Geometry check sheet. Reference: the model listing, model coordinates, mm. Face numbers are marked on the shaded views. A direction names the side the tool comes from. Coordinates: 2 decimals unless noted, no trailing zeros. Loops run counter-clockwise (first coordinate to the right, second up) from the corner with the lowest first, then second, coordinate; pieces in that order, holes last. Notation, with made-up numbers: M -9,-37.5 L 42,-37.5 A27 cw 42,-12.5 Z; hole C 15.5,54 d1. An arc over 180 degrees is marked long. Use CSV: the item, a comma, the result in double quotes.
Autodesk Inventor part; units mm, degrees
ref_plane "YZ Plane" through (0, 0, 0) normal (1, 0, 0) x (0, 1, 0)
ref_plane "XZ Plane" through (0, 0, 0) normal (0, 1, 0) x (-1, 0, 0)
ref_plane "XY Plane" through (0, 0, 0) normal (0, 0, 1) x (1, 0, 0)
sketch "Sketch1" plane through (0, 0, 0) normal (0, 0, 1) x (1, 0, 0)
  line L0 (0, 0) -> (22, 0)
  line L1 (22, 0) -> (22, -29)
  line L2 (22, -29) -> (0, -29)
  line L3 (0, -29) -> (0, 0)
  line L4 (3, -5.35) -> (19, -5.35)
  line L5 (19, -5.35) -> (19, -7.65)
  line L6 (19, -7.65) -> (3, -7.65)
  line L7 (3, -7.65) -> (3, -5.35)
  line L8 (3, -13.35) -> (19, -13.35)
  line L9 (19, -13.35) -> (19, -15.65)
  line L10 (19, -15.65) -> (3, -15.65)
  line L11 (3, -15.65) -> (3, -13.35)
  line L12 (3, -21.35) -> (19, -21.35)
  line L13 (19, -21.35) -> (19, -23.65)
  line L14 (19, -23.65) -> (3, -23.65)
  line L15 (3, -23.65) -> (3, -21.35)
  line L16 (19, -5.35) -> (19, -13.35) construction
  line L17 (19, -13.35) -> (19, -21.35) construction
  line L18 (22, -14.5) -> (0, -14.5) construction
  line L19 (11, 0) -> (11, -29) construction
  point P0 (19, -14.5)
  point P1 (11, -5.35)
  dimension "d0" = 22
  dimension "d1" = 29
  dimension "d2" = 2.3
  dimension "d3" = 8
  dimension "d4" = 16
extrude "Body with light pipe slots" add sketch "Sketch1" along normal blind 4.5
sketch "Sketch2" plane through (0, 0, 4.5) normal (0, 0, 1) x (1, 0, 0)
  line L0 (0, -29) -> (22, -29) construction
  line L1 (22, -29) -> (22, 0) construction
  line L2 (22, 0) -> (0, 0) construction
  line L3 (0, 0) -> (0, -29) construction
  line L4 (3, -21.35) -> (19, -21.35) construction
  line L5 (19, -21.35) -> (19, -23.65) construction
  line L6 (19, -23.65) -> (3, -23.65) construction
  line L7 (3, -23.65) -> (3, -21.35) construction
  line L8 (3, -13.35) -> (19, -13.35) construction
  line L9 (19, -13.35) -> (19, -15.65) construction
  line L10 (19, -15.65) -> (3, -15.65) construction
  line L11 (3, -15.65) -> (3, -13.35) construction
  line L12 (3, -5.35) -> (19, -5.35) construction
  line L13 (19, -5.35) -> (19, -7.65) construction
  line L14 (19, -7.65) -> (3, -7.65) construction
  line L15 (3, -7.65) -> (3, -5.35) construction
  line L16 (1, -5.35) -> (21, -5.35)
  line L17 (21, -5.35) -> (21, -7.65)
  line L18 (21, -7.65) -> (1, -7.65)
  line L19 (1, -7.65) -> (1, -5.35)
  line L20 (1, -13.35) -> (21, -13.35)
  line L21 (21, -13.35) -> (21, -15.65)
  line L22 (21, -15.65) -> (1, -15.65)
  line L23 (1, -15.65) -> (1, -13.35)
  line L24 (1, -21.35) -> (21, -21.35)
  line L25 (21, -21.35) -> (21, -23.65)
  line L26 (21, -23.65) -> (1, -23.65)
  line L27 (1, -23.65) -> (1, -21.35)
  dimension "d7" = 2
  dimension "d8" = 2
extrude "Light pipe wing cuts" cut sketch "Sketch2" against normal blind 4
sketch "Sketch3" plane through (0, 0, 4.5) normal (0, 0, 1) x (1, 0, 0)
  line L0 (1, -21.35) -> (21, -21.35) construction
  line L1 (21, -21.35) -> (21, -23.65) construction
  line L2 (21, -23.65) -> (1, -23.65) construction
  line L3 (1, -23.65) -> (1, -21.35) construction
  line L4 (1, -13.35) -> (21, -13.35) construction
  line L5 (21, -13.35) -> (21, -15.65) construction
  line L6 (21, -15.65) -> (1, -15.65) construction
  line L7 (1, -15.65) -> (1, -13.35) construction
  line L8 (1, -5.35) -> (21, -5.35) construction
  line L9 (21, -5.35) -> (21, -7.65) construction
  line L10 (21, -7.65) -> (1, -7.65) construction
  line L11 (1, -7.65) -> (1, -5.35) construction
  line L12 (0, -29) -> (22, -29) construction
  line L13 (22, -29) -> (22, 0) construction
  line L14 (22, 0) -> (0, 0) construction
  line L15 (0, 0) -> (0, -29) construction
  line L16 (3, -5.35) -> (3, -7.65) construction
  line L17 (19, -7.65) -> (19, -5.35) construction
  line L18 (19, -15.65) -> (19, -13.35) construction
  line L19 (19, -23.65) -> (19, -21.35) construction
  line L20 (3, -21.35) -> (3, -23.65) construction
  line L21 (3, -13.35) -> (3, -15.65) construction
  line L22 (3, -4.35) -> (19, -4.35)
  line L23 (19, -4.35) -> (19, -8.65)
  line L24 (19, -8.65) -> (3, -8.65)
  line L25 (3, -8.65) -> (3, -4.35)
  line L26 (3, -12.35) -> (19, -12.35)
  line L27 (19, -12.35) -> (19, -16.65)
  line L28 (19, -16.65) -> (3, -16.65)
  line L29 (3, -16.65) -> (3, -12.35)
  line L30 (3, -20.2545) -> (19, -20.2545)
  line L31 (19, -20.2545) -> (19, -24.5545)
  line L32 (19, -24.5545) -> (3, -24.5545)
  line L33 (3, -24.5545) -> (3, -20.2545)
  dimension "d11" = 1
  dimension "d12" = 1
  dimension "d13" = 1.0956
  dimension "d14" = 1
extrude "SMD clearance cuts" cut sketch "Sketch3" against normal blind 1
sketch "Sketch4" plane through (0, 0, 0) normal (0, 0, -1) x (-1, 0, 0)
  line L0 (-22, 0) -> (0, 0) construction
  line L1 (-11, 0) -> (-11, -29) construction
  line L2 (0, -29) -> (-22, -29) construction
  line L3 (-12, -2.15) -> (-10, -2.15)
  line L4 (-10, -26.85) -> (-12, -26.85)
  line L5 (-3, -5.35) -> (-19, -5.35)
  line L6 (-19, -23.65) -> (-3, -23.65)
  line L7 (-6.75, -23.65) -> (-6.75, -25.15)
  line L8 (-15.25, -25.15) -> (-15.25, -23.65)
  line L9 (-19, -15.65) -> (-3, -15.65)
  line L10 (-6.75, -15.65) -> (-6.75, -17.15)
  line L11 (-15.25, -17.15) -> (-15.25, -15.65)
  line L12 (-3, -7.65) -> (-19, -7.65)
  line L13 (-6.75, -7.65) -> (-6.75, -9.15)
  line L14 (-15.25, -9.15) -> (-15.25, -7.65)
  line L15 (-12, -7.65) -> (-12, -2.15)
  line L16 (-10, -2.15) -> (-10, -7.65)
  line L17 (-6.75, -9.15) -> (-10, -9.15)
  line L18 (-12, -9.15) -> (-15.25, -9.15)
  line L19 (-12, -15.65) -> (-12, -9.15)
  line L20 (-10, -9.15) -> (-10, -15.65)
  line L21 (-15.25, -15.65) -> (-12, -15.65)
  line L22 (-10, -15.65) -> (-6.75, -15.65)
  line L23 (-6.75, -17.15) -> (-10, -17.15)
  line L24 (-12, -17.15) -> (-15.25, -17.15)
  line L25 (-15.25, -23.65) -> (-12, -23.65)
  line L26 (-10, -23.65) -> (-6.75, -23.65)
  line L27 (-6.75, -25.15) -> (-10, -25.15)
  line L28 (-12, -25.15) -> (-15.25, -25.15)
  line L29 (-12, -26.85) -> (-12, -25.15)
  line L30 (-12, -23.65) -> (-12, -17.15)
  line L31 (-10, -17.15) -> (-10, -23.65)
  line L32 (-10, -25.15) -> (-10, -26.85)
  line L33 (-15.25, -7.65) -> (-12, -7.65)
  line L34 (-10, -7.65) -> (-6.75, -7.65)
  point P0 (-11, -2.15)
  dimension "d17" = 3.2
  dimension "d18" = 2
  dimension "d19" = 3.2
  dimension "d20" = 1.5
  dimension "d21" = 8.5
  dimension "d22" = 4.25
extrude "Case interior molding cuts" cut sketch "Sketch4" against normal blind 3
equation "\"d8\" = d7"
equation "\"d12\" = d11"
equation "\"d14\" = d11"
equation "\"d22\" = 0.5 * d21"
properties part number "Lightpipe shield"
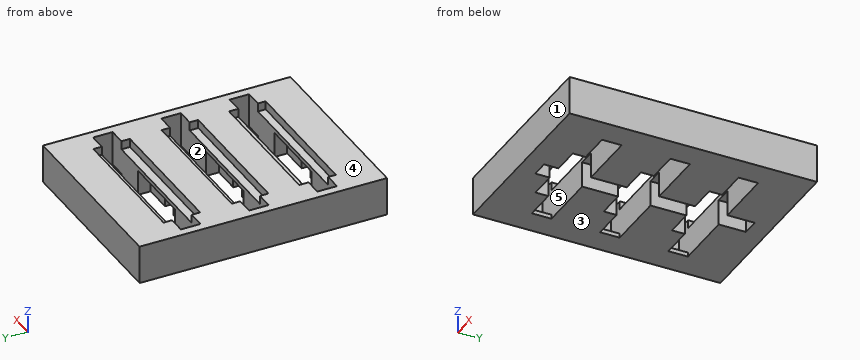
1. Gauge pin test, flat ends, axial feed: P1, Ø6, axis at x = 9.5, y = -8, coming from the -Z side; P2, Ø0.6, axis at x = 1.5, y = -14, coming from the +Z side. Record the tip position at first contact, or that the pin passes through.
The answers:
P1,"z = 0"
P2,"z = 0.5"
2. Section check A-A, the plane x = 12.75. Count the separate pieces of the cut face and the enclosed holes in it, plus the area to 4 significant figures.
The answers:
separate pieces,"4"
enclosed holes,"0"
area,"79.95 mm^2"
3. Thickness scan on line 1 (Y direction, x = 16.75, z = 0.9); line 2 (X direction, y = -25.5, z = 1.2); line 3 (Y direction, x = 13.5, z = 0.5). Record the ranges inside material, lowest first. Write a range as [from, to].
The answers:
line 1,"[-29, -23.65], [-21.35, -15.65], [-13.35, -7.65], [-5.35, 0]"
line 2,"[0, 10], [12, 22]"
line 3,"[-29, -25.15], [-21.35, -17.15], [-13.35, -9.15], [-5.35, 0]"
4. Set-up check for the marked faces 4 and 5: record each of +Z, -Z, +X, -X, +Y, -Y from which the full face is reachable in a straight line by a thin tool's end or side.
The answers:
face 4,"+Z, +X, -X, +Y, -Y"
face 5,"+Z"
5. Section check D-D, the plane y = -8.25. Record the cut outline in (x, z), plus the area to 3 significant figures.
The answers:
outline,"M 0,0 L 6.75,0 L 6.75,3 L 15.25,3 L 15.25,0 L 22,0 L 22,4.5 L 19,4.5 L 19,3.5 L 3,3.5 L 3,4.5 L 0,4.5 Z"
area,"57.5 mm^2"
6. Section check C-C, the plane x = 18. Record the cut outline in (y, z).
The answers:
outline,"M -29,0 L -23.65,0 L -23.65,3.5 L -24.55,3.5 L -24.55,4.5 L -29,4.5 Z; M -21.35,0 L -15.65,0 L -15.65,3.5 L -16.65,3.5 L -16.65,4.5 L -20.25,4.5 L -20.25,3.5 L -21.35,3.5 Z; M -13.35,0 L -7.65,0 L -7.65,3.5 L -8.65,3.5 L -8.65,4.5 L -12.35,4.5 L -12.35,3.5 L -13.35,3.5 Z; M -5.35,0 L 0,0 L 0,4.5 L -4.35,4.5 L -4.35,3.5 L -5.35,3.5 Z"
7. Section check B-B, the plane y = -14. Record the cut outline in (x, z).
The answers:
outline,"M 0,0 L 3,0 L 3,0.5 L 1,0.5 L 1,4.5 L 0,4.5 Z; M 19,0 L 22,0 L 22,4.5 L 21,4.5 L 21,0.5 L 19,0.5 Z"
8. Release check for a two-part mould opening along Y. For the marked faces 1, 2 and 3 record: +Y half, -Y half, draft (parallel to the pull), parting line (faces both ways), or undercut.
The answers:
face 1,"-Y half"
face 2,"undercut"
face 3,"draft"
